Work out the finished part from the listing and answer in its coordinate system (mm). A direction names the side the tool comes from. Give positions to 0.01 mm unless a question says otherwise; leave off trailing zeros. Order: outer loops, then holes, each group sorted by start corner. A loop starts at its lowest first (then second) coordinate and runs counter-clockwise, first axis right, second up. Notation, with made-up numbers: (-9.75, 9) - (48.25, 9) arc R14 cw to (48.25, 19) - close; hole circle Ø1 at (9, 83). An arc over 180 degrees is marked (long way). Return JSON: item names as keys, results as strings. Group by question number.
from build123d import *

# Parameters (mm, degrees)
SKETCH_1_W                = 60
SKETCH_1_H                = 60
EXTRUDE_1_DEPTH           = 55.5
SKETCH_2_W                = 50
SKETCH_2_H                = 50
CUT_EXTRUDE_3_DEPTH       = 49.5
SKETCH_4_W                = 38.4
SKETCH_4_H                = 38.4
CUT_EXTRUDE_4_DEPTH       = 4
SKETCH_5_W                = 8
SKETCH_5_H                = 8
EXTRUDE_3_DEPTH           = 2.5
CUT_EXTRUDE_5_REACH       = 56
SKETCH_6_R                = 1.25
SKETCH_7_R                = 11.5
CUT_EXTRUDE_6_DEPTH       = 2.5
FILLET_5_R                = 1
SKETCH_12_W               = 60
SKETCH_12_H               = 60
CUT_EXTRUDE_9_DEPTH       = 3
SKETCH_17_W               = 60
SKETCH_17_H               = 60
EXTRUDE_5_DEPTH           = 13.5
SKETCH_20_W               = 54
SKETCH_20_H               = 54
EXTRUDE_6_DEPTH           = 6
SKETCH_21_W               = 46
SKETCH_21_H               = 46
CUT_EXTRUDE_18_DEPTH      = 6
FILLET_9_R                = 2
FILLET_10_R               = 2
SKETCH_24_W               = 52
SKETCH_24_H               = 52
CUT_EXTRUDE_21_DEPTH      = 13.5
CUT_EXTRUDE_22_REACH      = 62
SKETCH_25_W               = 7
SKETCH_25_H               = 20
EXTRUDE_7_DEPTH           = 4.5
SKETCH_27_W               = 52
SKETCH_27_H               = 52
CUT_EXTRUDE_24_DEPTH      = 4.5
SKETCH_28_W               = 7
SKETCH_28_H               = 24
CUT_EXTRUDE_25_DEPTH      = 4.5
CUT_EXTRUDE_26_REACH      = 74
SKETCH_29_R               = 2.1
FILLET_12_R               = 2
SKETCH_30_R               = 1.5
CUT_EXTRUDE_27_DEPTH      = 24
CUT_EXTRUDE_27_DEPTH_BACK = 78
SKETCH_31_R               = 1.5
CUT_EXTRUDE_28_DEPTH      = 24
CUT_EXTRUDE_28_DEPTH_BACK = 78
FILLET_13_R               = 2
FILLET_14_R               = 2


with BuildPart() as part:
    # 草图1 → 凸台-拉伸1 (new body)
    with BuildSketch(Plane.XY):
        Rectangle(SKETCH_1_W, SKETCH_1_H)
    extrude(amount=EXTRUDE_1_DEPTH)

    # 草图2 → 切除-拉伸3 (cut)
    with BuildSketch(Plane.XY.offset(55.5)):
        Rectangle(SKETCH_2_W, SKETCH_2_H)
    extrude(amount=-CUT_EXTRUDE_3_DEPTH, mode=Mode.SUBTRACT)

    # 草图4 → 切除-拉伸4 (cut)
    with BuildSketch(Plane(origin=(0, 0, 0), x_dir=(-1, 0, 0), z_dir=(0, 0, -1))):
        Rectangle(SKETCH_4_W, SKETCH_4_H)
    extrude(amount=-CUT_EXTRUDE_4_DEPTH, mode=Mode.SUBTRACT)

    # 草图5 → 凸台-拉伸3 (add)
    with BuildSketch(Plane(origin=(0, 0, 4), x_dir=(-1, 0, 0), z_dir=(0, 0, -1))):
        with Locations((-15.2, 15.2)):
            Rectangle(SKETCH_5_W, SKETCH_5_H)
        with Locations((15.2, 15.2)):
            Rectangle(SKETCH_5_W, SKETCH_5_H)
        with Locations((15.2, -15.2)):
            Rectangle(SKETCH_5_W, SKETCH_5_H)
        with Locations((-15.2, -15.2)):
            Rectangle(SKETCH_5_W, SKETCH_5_H)
    extrude(amount=EXTRUDE_3_DEPTH)

    # 草图6 → 切除-拉伸5 (cut, up to next)
    with BuildSketch(Plane(origin=(0, 0, 1.5), x_dir=(-1, 0, 0), z_dir=(0, 0, -1)), mode=Mode.PRIVATE) as cut_extrude_5_sk1:
        with Locations((-14, 14)):
            Circle(SKETCH_6_R)
    cut_extrude_5_tool1 = extrude(cut_extrude_5_sk1.sketch, amount=-CUT_EXTRUDE_5_REACH, mode=Mode.PRIVATE) & part.part
    add(cut_extrude_5_tool1.solids().sort_by_distance((14, 14, 1.5))[0], mode=Mode.SUBTRACT)
    # 草图6 → 切除-拉伸5 (cut, up to next)
    with BuildSketch(Plane(origin=(0, 0, 1.5), x_dir=(-1, 0, 0), z_dir=(0, 0, -1)), mode=Mode.PRIVATE) as cut_extrude_5_sk2:
        with Locations((14, 14)):
            Circle(SKETCH_6_R)
    cut_extrude_5_tool2 = extrude(cut_extrude_5_sk2.sketch, amount=-CUT_EXTRUDE_5_REACH, mode=Mode.PRIVATE) & part.part
    add(cut_extrude_5_tool2.solids().sort_by_distance((-14, 14, 1.5))[0], mode=Mode.SUBTRACT)
    # 草图6 → 切除-拉伸5 (cut, up to next)
    with BuildSketch(Plane(origin=(0, 0, 1.5), x_dir=(-1, 0, 0), z_dir=(0, 0, -1)), mode=Mode.PRIVATE) as cut_extrude_5_sk3:
        with Locations((-14, -14)):
            Circle(SKETCH_6_R)
    cut_extrude_5_tool3 = extrude(cut_extrude_5_sk3.sketch, amount=-CUT_EXTRUDE_5_REACH, mode=Mode.PRIVATE) & part.part
    add(cut_extrude_5_tool3.solids().sort_by_distance((14, -14, 1.5))[0], mode=Mode.SUBTRACT)
    # 草图6 → 切除-拉伸5 (cut, up to next)
    with BuildSketch(Plane(origin=(0, 0, 1.5), x_dir=(-1, 0, 0), z_dir=(0, 0, -1)), mode=Mode.PRIVATE) as cut_extrude_5_sk4:
        with Locations((13.997534232, -14.034417217)):
            Circle(SKETCH_6_R)
    cut_extrude_5_tool4 = extrude(cut_extrude_5_sk4.sketch, amount=-CUT_EXTRUDE_5_REACH, mode=Mode.PRIVATE) & part.part
    add(cut_extrude_5_tool4.solids().sort_by_distance((-13.997534, -14.034417, 1.5))[0], mode=Mode.SUBTRACT)

    # 草图7 → 切除-拉伸6 (cut)
    with BuildSketch(Plane(origin=(0, 0, 4), x_dir=(-1, 0, 0), z_dir=(0, 0, -1))):
        Circle(SKETCH_7_R)
    extrude(amount=-CUT_EXTRUDE_6_DEPTH, mode=Mode.SUBTRACT)

    # 圆角5
    fillet_5_edges = [part.edges().sort_by_distance(p)[0] for p in [
        (19.2, 11.2, 2.75),
        (11.2, 11.2, 2.75),
        (11.2, 19.2, 2.75),
        (-19.2, 11.2, 2.75),
        (-11.2, 19.2, 2.75),
        (-11.2, 11.2, 2.75),
        (-19.2, -11.2, 2.75),
        (-11.2, -11.2, 2.75),
        (-11.2, -19.2, 2.75),
        (19.2, -11.2, 2.75),
        (11.2, -19.2, 2.75),
        (11.2, -11.2, 2.75),
    ]]
    fillet(fillet_5_edges, radius=FILLET_5_R)

    # 草图12 → 切除-拉伸9 (cut)
    with BuildSketch(Plane.XY.offset(55.5)):
        Rectangle(SKETCH_12_W, SKETCH_12_H)
    extrude(amount=-CUT_EXTRUDE_9_DEPTH, mode=Mode.SUBTRACT)

    # 草图17 → 凸台-拉伸5 (add)
    with BuildSketch(Plane(origin=(0, 0, 0), x_dir=(-1, 0, 0), z_dir=(0, 0, -1))):
        Rectangle(SKETCH_17_W, SKETCH_17_H)
    extrude(amount=EXTRUDE_5_DEPTH)

    # 草图20 → 凸台-拉伸6 (add)
    with BuildSketch(Plane.XY.offset(52.5)):
        Rectangle(SKETCH_20_W, SKETCH_20_H)
    extrude(amount=EXTRUDE_6_DEPTH)

    # 草图21 → 切除-拉伸18 (cut)
    with BuildSketch(Plane.XY.offset(58.5)):
        Rectangle(SKETCH_21_W, SKETCH_21_H)
    extrude(amount=-CUT_EXTRUDE_18_DEPTH, mode=Mode.SUBTRACT)

    # 圆角9
    fillet_9_edges = [part.edges().sort_by_distance(p)[0] for p in [
        (25, 25, 29.25),
        (25, -25, 29.25),
        (-25, -25, 29.25),
        (-25, 25, 29.25),
        (23, 23, 55.5),
        (23, -23, 55.5),
        (-23, -23, 55.5),
        (-23, 23, 55.5),
    ]]
    fillet(fillet_9_edges, radius=FILLET_9_R)

    # 圆角10
    fillet_10_edges = [part.edges().sort_by_distance(p)[0] for p in [
        (-27, -27, 55.5),
        (27, -27, 55.5),
        (27, 27, 55.5),
        (-27, 27, 55.5),
    ]]
    fillet(fillet_10_edges, radius=FILLET_10_R)

    # 草图24 → 切除-拉伸21 (cut)
    with BuildSketch(Plane(origin=(0, 0, -13.5), x_dir=(-1, 0, 0), z_dir=(0, 0, -1))):
        Rectangle(SKETCH_24_W, SKETCH_24_H)
    extrude(amount=-CUT_EXTRUDE_21_DEPTH, mode=Mode.SUBTRACT)

    # 草图25 → 切除-拉伸22 (cut, up to next)
    with BuildSketch(Plane(origin=(0, 30, 0), x_dir=(1, 0, 0), z_dir=(0, 1, 0)), mode=Mode.PRIVATE) as cut_extrude_22_sk1:
        with Locations((0, 13.5)):
            Rectangle(SKETCH_25_W, SKETCH_25_H)
    cut_extrude_22_tool1 = extrude(cut_extrude_22_sk1.sketch, amount=-CUT_EXTRUDE_22_REACH, mode=Mode.PRIVATE) & part.part
    add(cut_extrude_22_tool1.solids().sort_by_distance((0, 30, -13.5))[0], mode=Mode.SUBTRACT)

    # 草图26 → 凸台-拉伸7 (add)
    with BuildSketch(Plane(origin=(0, 0, -13.5), x_dir=(-1, 0, 0), z_dir=(0, 0, -1))):
        Polygon((-31.5, -50), (-50, -50), (-50, 31.5), (-50, 50), (30, 50), (50, 50), (50, -31.5), (50, -50), align=None)
    extrude(amount=-EXTRUDE_7_DEPTH)

    # 草图27 → 切除-拉伸24 (cut)
    with BuildSketch(Plane(origin=(0, 0, -13.5), x_dir=(-1, 0, 0), z_dir=(0, 0, -1))):
        Rectangle(SKETCH_27_W, SKETCH_27_H)
    extrude(amount=-CUT_EXTRUDE_24_DEPTH, mode=Mode.SUBTRACT)

    # 草图28 → 切除-拉伸25 (cut)
    with BuildSketch(Plane(origin=(0, 0, -13.5), x_dir=(-1, 0, 0), z_dir=(0, 0, -1))):
        with Locations((0, 38)):
            Rectangle(SKETCH_28_W, SKETCH_28_H)
    extrude(amount=-CUT_EXTRUDE_25_DEPTH, mode=Mode.SUBTRACT)

    # 草图29 → 切除-拉伸26 (cut, up to next)
    with BuildSketch(Plane(origin=(0, 0, -13.5), x_dir=(-1, 0, 0), z_dir=(0, 0, -1)), mode=Mode.PRIVATE) as cut_extrude_26_sk1:
        with Locations((-40, 40)):
            Circle(SKETCH_29_R)
    cut_extrude_26_tool1 = extrude(cut_extrude_26_sk1.sketch, amount=-CUT_EXTRUDE_26_REACH, mode=Mode.PRIVATE) & part.part
    add(cut_extrude_26_tool1.solids().sort_by_distance((40, 40, -13.5))[0], mode=Mode.SUBTRACT)
    # 草图29 → 切除-拉伸26 (cut, up to next)
    with BuildSketch(Plane(origin=(0, 0, -13.5), x_dir=(-1, 0, 0), z_dir=(0, 0, -1)), mode=Mode.PRIVATE) as cut_extrude_26_sk2:
        with Locations((40, 40)):
            Circle(SKETCH_29_R)
    cut_extrude_26_tool2 = extrude(cut_extrude_26_sk2.sketch, amount=-CUT_EXTRUDE_26_REACH, mode=Mode.PRIVATE) & part.part
    add(cut_extrude_26_tool2.solids().sort_by_distance((-40, 40, -13.5))[0], mode=Mode.SUBTRACT)
    # 草图29 → 切除-拉伸26 (cut, up to next)
    with BuildSketch(Plane(origin=(0, 0, -13.5), x_dir=(-1, 0, 0), z_dir=(0, 0, -1)), mode=Mode.PRIVATE) as cut_extrude_26_sk3:
        with Locations((40, -40)):
            Circle(SKETCH_29_R)
    cut_extrude_26_tool3 = extrude(cut_extrude_26_sk3.sketch, amount=-CUT_EXTRUDE_26_REACH, mode=Mode.PRIVATE) & part.part
    add(cut_extrude_26_tool3.solids().sort_by_distance((-40, -40, -13.5))[0], mode=Mode.SUBTRACT)
    # 草图29 → 切除-拉伸26 (cut, up to next)
    with BuildSketch(Plane(origin=(0, 0, -13.5), x_dir=(-1, 0, 0), z_dir=(0, 0, -1)), mode=Mode.PRIVATE) as cut_extrude_26_sk4:
        with Locations((-40, -40)):
            Circle(SKETCH_29_R)
    cut_extrude_26_tool4 = extrude(cut_extrude_26_sk4.sketch, amount=-CUT_EXTRUDE_26_REACH, mode=Mode.PRIVATE) & part.part
    add(cut_extrude_26_tool4.solids().sort_by_distance((40, -40, -13.5))[0], mode=Mode.SUBTRACT)

    # 圆角12
    fillet_12_edges = [part.edges().sort_by_distance(p)[0] for p in [
        (-30, -30, 21.75),
        (-30, 30, 21.75),
        (30, 30, 21.75),
        (30, -30, 21.75),
    ]]
    fillet(fillet_12_edges, radius=FILLET_12_R)

    # 草图30 → 切除-拉伸27 (cut, two sides)
    with BuildSketch(Plane.ZY.offset(27)) as cut_extrude_27_sk:
        with Locations((55.5, 0)):
            Circle(SKETCH_30_R)
    extrude(amount=CUT_EXTRUDE_27_DEPTH, mode=Mode.SUBTRACT)
    extrude(cut_extrude_27_sk.sketch, amount=-CUT_EXTRUDE_27_DEPTH_BACK, mode=Mode.SUBTRACT)

    # 草图31 → 切除-拉伸28 (cut, two sides)
    with BuildSketch(Plane(origin=(0, 27, 0), x_dir=(1, 0, 0), z_dir=(0, 1, 0))) as cut_extrude_28_sk:
        with Locations((0, -55.5)):
            Circle(SKETCH_31_R)
    extrude(amount=CUT_EXTRUDE_28_DEPTH, mode=Mode.SUBTRACT)
    extrude(cut_extrude_28_sk.sketch, amount=-CUT_EXTRUDE_28_DEPTH_BACK, mode=Mode.SUBTRACT)

    # 圆角13
    fillet_13_edges = [part.edges().sort_by_distance(p)[0] for p in [
        (-26, 26, -6.75),
        (-26, -26, -6.75),
        (26, -26, -6.75),
        (26, 26, -6.75),
    ]]
    fillet(fillet_13_edges, radius=FILLET_13_R)

    # 圆角14
    fillet_14_edges = [part.edges().sort_by_distance(p)[0] for p in [
        (50, -50, -11.25),
        (50, 50, -11.25),
        (-50, 50, -11.25),
        (-50, -50, -11.25),
    ]]
    fillet(fillet_14_edges, radius=FILLET_14_R)


solid = part.part
1. A tool of negligible diameter and unlimited length cuts with its end or side. For faces 1 (the flat face through (30, 0, 22)), 2 (the flat face through (-2, -24, 52.5)), 3 (the flat face through (0, 29, 52.5)), 4 (the flat face through (-30, 0, 22)), 5 (the flat face through (15, -11.2, 3)), from which of +Z, -Z, +X, -X, +Y, -Y can it reach the whole face along a straight path? Write none if from no direction.
2. The part is cut by section B-B (z = 55.5). State how many separate pieces and enclosed holes the cut face has, and give its area (3 significant figures).
3. Consider probe 1 along Y at (x, z) = (40, -10); probe 2 along X at (y, z) = (-11, 43.5). Determine where each line is inside the solid, lowest interval first. Write a range as from..to.
4. The part is cut by section D-D (z = 8.5). Give the vertices of the cut face in (x, y), and give its area (3 significant figures).
5. Determine the mould class of faces 6 (the flat face through (0, 27, 53)), 7 (the flat face through (-16, -16, 1.5)), 8 (the flat face through (-25, 0, 30)) for opening direction Z: released by +Z, released by -Z, zero draft, split by the parting line, or undercut.
6. The part is cut by section C-C (y = 40). Give the vertices of the cut face in (x, z).
7. The part is cut by section A-A (y = -40). Give the vertices of the cut face in (x, z).
8. Each of these flat-tipped pins is pushed along its axis until it touches: pin 1 (1.2 mm diameter, centred on y = -14, z = 3, fed in from -X); pin 2 (6.5 mm diameter, centred on y = -6, z = 54.5, fed in from +X); pin 3 (1.2 mm diameter, centred on x = -15, z = 2.5, fed in from -Y); pin 4 (2.5 mm diameter, centred on x = 0, z = 55.5, fed in from +Y) (3 decimals). Where does it stop, or does it pass through?
Answers:
{
 "1": {"face 1": "+Z, +X, +Y, -Y", "face 2": "none", "face 3": "+Z", "face 4": "+Z, -X, +Y, -Y", "face 5": "-Z"},
 "2": {"separate pieces": "4", "enclosed holes": "0", "area": "752 mm^2"},
 "3": {"probe 1": "y = -50..-42.1, -37.9..37.9, 42.1..50", "probe 2": "x = -30..-25, 25..30"},
 "4": {"outline": "(-30, -28) arc R2 ccw to (-28, -30) - (28, -30) arc R2 ccw to (30, -28) - (30, 28) arc R2 ccw to (28, 30) - (-28, 30) arc R2 ccw to (-30, 28) - close; hole (-25, -23) arc R2 ccw to (-23, -25) - (23, -25) arc R2 ccw to (25, -23) - (25, 23) arc R2 ccw to (23, 25) - (-23, 25) arc R2 ccw to (-25, 23) - close", "area": "1,100 mm^2"},
 "5": {"face 6": "zero draft", "face 7": "released by -Z", "face 8": "undercut"},
 "6": {"outline": "(-50, -13.5) - (-42.1, -13.5) - (-42.1, -9) - (-50, -9) - close; (-37.9, -13.5) - (-3.5, -13.5) - (-3.5, -9) - (-37.9, -9) - close; (3.5, -13.5) - (37.9, -13.5) - (37.9, -9) - (3.5, -9) - close; (42.1, -13.5) - (50, -13.5) - (50, -9) - (42.1, -9) - close"},
 "7": {"outline": "(-50, -13.5) - (-42.1, -13.5) - (-42.1, -9) - (-50, -9) - close; (-37.9, -13.5) - (37.9, -13.5) - (37.9, -9) - (-37.9, -9) - close; (42.1, -13.5) - (50, -13.5) - (50, -9) - (42.1, -9) - close"},
 "8": {"pin 1": "stops at x = -30", "pin 2": "stops at x = 30", "pin 3": "stops at y = -30", "pin 4": "passes through"}
}
